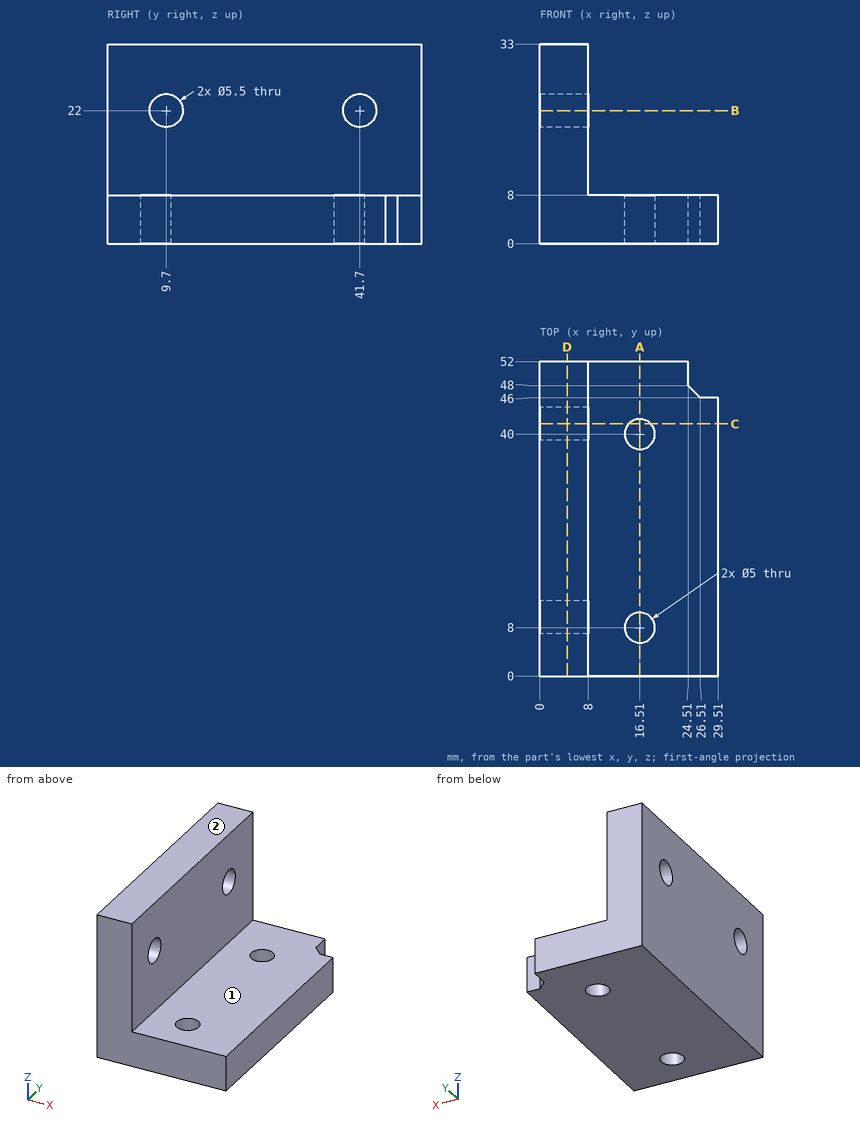
Source: three-view drawing plus pictorial views. Frame: mm from the lowest corner of the part. A direction names the side the tool comes from. Give positions to 0.01 mm unless a question says otherwise; leave off trailing zeros. Loops run counter-clockwise (first coordinate to the right, second up) from the corner with the lowest first, then second, coordinate; pieces in that order, holes last.
1) Section query C-C on y = 41.7. Return the cut outline in (x, z).
A:
outline: (0, 0) - (14.68, 0) - (14.68, 8) - (8, 8) - (8, 19.25) - (0, 19.25) - close; (0, 24.75) - (8, 24.75) - (8, 33) - (0, 33) - close; (18.34, 0) - (29.51, 0) - (29.51, 8) - (18.34, 8) - close
2) Section query A-A on x = 16.51. Return the cut outline in (y, z), and give its area (3 significant figures).
A:
outline: (0, 0) - (5.5, 0) - (5.5, 8) - (0, 8) - close; (10.5, 0) - (37.5, 0) - (37.5, 8) - (10.5, 8) - close; (42.5, 0) - (52, 0) - (52, 8) - (42.5, 8) - close
area: 336 mm2
3) Section query D-D on x = 4.5. Return the cut outline in (y, z).
A:
outline: (0, 0) - (52, 0) - (52, 33) - (0, 33) - close; hole circle Ø5.5 at (9.7, 22); hole circle Ø5.5 at (41.7, 22)
4) Section query B-B on z = 22. Return the cut outline in (x, y).
A:
outline: (0, 0) - (8, 0) - (8, 6.95) - (0, 6.95) - close; (0, 12.45) - (8, 12.45) - (8, 38.95) - (0, 38.95) - close; (0, 44.45) - (8, 44.45) - (8, 52) - (0, 52) - close
5) Contact query for flat-ended pins moving along their axis: pin 1 (6.5 mm diameter, centred on y = 41.7, z = 22, fed in from +X); pin 2 (2 mm diameter, centred on y = 50.5, z = 2, fed in from +X); pin 3 (17 mm diameter, centred on x = 18.5, y = 36, fed in from +Z). Output: stop coordinate, or through.
A:
pin 1: stops at x = 8
pin 2: stops at x = 24.51
pin 3: stops at z = 8
6) Line query: L1, parallel to Y at x = 6, z = 22; L2, parallel to X at y = 24, z = 14.5; L3, parallel to Z at x = 3.75, y = 44. Output: solid intervals per line, ascending.
A:
L1: y = 0 to 6.95, 12.45 to 38.95, 44.45 to 52
L2: x = 0 to 8
L3: z = 0 to 20.49, 23.51 to 33
7) Reachability of the marked faces 1 and 2 from +Z, -Z, +X, -X, +Y, -Y: full face, straight path, thin tool, end or side. Return the list, or none.
A:
face 1: +Z, +X, +Y, -Y
face 2: +Z, +X, -X, +Y, -Y
